from build123d import *

# Parameters (mm, degrees)
F0_W     = 28.448
F0_H     = 2.032
F0_W_2   = 2.032
F0_H_2   = 23.368
F1_DEPTH = 50.8
F2_R     = 2.54
F3_R     = 1.778
F5_D     = 3.81


with BuildPart() as f1:
    # F0 (on Front) → F1 (new body, symmetric)
    with BuildSketch(Plane.XZ):
        with Locations((-39.1122124221, 13.9883446444)):
            Rectangle(F0_W, F0_H)
        with Locations((-54.3522124221, 13.9883446444)):
            Rectangle(F0_W_2, F0_H)
        with Locations((-54.3522124221, 26.6883446444)):
            Rectangle(F0_W_2, F0_H_2)
    extrude(amount=F1_DEPTH, both=True)

    # F2
    f2_edges = [f1.edges().sort_by_distance(p)[0] for p in [
        (-55.368212, 0, 12.972345),
    ]]
    fillet(f2_edges, radius=F2_R)

    # F3
    f3_edges = [f1.edges().sort_by_distance(p)[0] for p in [
        (-53.336212, 0, 15.004345),
    ]]
    fillet(f3_edges, radius=F3_R)

    # F5 (through all)
    with Locations(Plane.YZ):
        with Locations((0, 34.6949249506), (0, 29.1896369308), (0, 24.1528842598)):
            Hole(F5_D / 2)


solid = f1.part
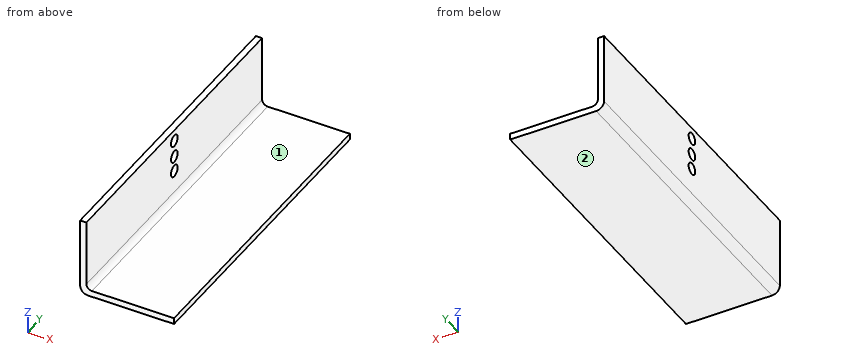
Geometry: final body of the model. Coordinates: model frame, mm. Face numbers are marked on the shaded views. A direction names the side the tool comes from. Give positions to 0.01 mm unless a question says otherwise; leave off trailing zeros. Write each loop counter-clockwise with the first axis right and the second up, starting at its lowest first coordinate (ties: lowest second). Pieces come first, ordered by that corner, then holes. Notation, with made-up numbers: (-18, 82) -> (-3, 82) arc R25 ccw to (-3, 102) -> close; hole circle Ø4 at (65, -13). An arc over 180 degrees is marked (long way). Answer in a Markdown table with one row per item.
(1) Section query B-B on y = -32.5. Return loops of the section in (x, z), then the cut area to 3 significant figures.
Answers below:
| item | result |
|---|---|
| outline | (-55.37, 15.51) arc R2.54 ccw to (-52.83, 12.97) -> (-24.89, 12.97) -> (-24.89, 15) -> (-51.56, 15) arc R1.78 cw to (-53.34, 16.78) -> (-53.34, 38.37) -> (-55.37, 38.37) -> close |
| area | 109 mm^2 |
(2) Ray query, line 1 along Z through (x, y) = (-54, 0); line 2 along Z through (x, y) = (-54.5, 0); line 3 along Z through (x, y) = (-28, 32). Return the intervals inside material, ascending. Write a range as [from, to].
Answers below:
| item | result |
|---|---|
| line 1 | [13.26, 22.25], [26.06, 27.28], [31.09, 32.79], [36.6, 38.37] |
| line 2 | [13.6, 22.25], [26.06, 27.28], [31.09, 32.79], [36.6, 38.37] |
| line 3 | [12.97, 15] |
(3) Section query A-A on y = 0. Return loops of the section in (x, z).
Answers below:
| item | result |
|---|---|
| outline | (-55.37, 15.51) arc R2.54 ccw to (-52.83, 12.97) -> (-24.89, 12.97) -> (-24.89, 15) -> (-51.56, 15) arc R1.78 cw to (-53.34, 16.78) -> (-53.34, 22.25) -> (-55.37, 22.25) -> close; (-55.37, 26.06) -> (-53.34, 26.06) -> (-53.34, 27.28) -> (-55.37, 27.28) -> close; (-55.37, 31.09) -> (-53.34, 31.09) -> (-53.34, 32.79) -> (-55.37, 32.79) -> close; (-55.37, 36.6) -> (-53.34, 36.6) -> (-53.34, 38.37) -> (-55.37, 38.37) -> close |
(4) Set-up query: the marked faces 1 and 2. Return all of +Z, -Z, +X, -X, +Y, -Y with unobstructed straight access to the full face (end or side cutting, diameter ignored); none if empty.
Answers below:
| item | result |
|---|---|
| face 1 | +Z, +X, +Y, -Y |
| face 2 | -Z, +X, -X, +Y, -Y |
(5) Pin query (flat end, axial travel): pin 1 (1.5 mm diameter, centred on y = 1.5, z = 32, fed in from +X); pin 2 (3.5 mm diameter, centred on y = 0, z = 29.19, fed in from +X). Return the tip coordinate at first contact, or that it passes through.
Answers below:
| item | result |
|---|---|
| pin 1 | x = -53.34 |
| pin 2 | through |
(6) Section query C-C on x = -46.5. Return loops of the section in (y, z).
Answers below:
| item | result |
|---|---|
| outline | (-50.8, 12.97) -> (50.8, 12.97) -> (50.8, 15) -> (-50.8, 15) -> close |
